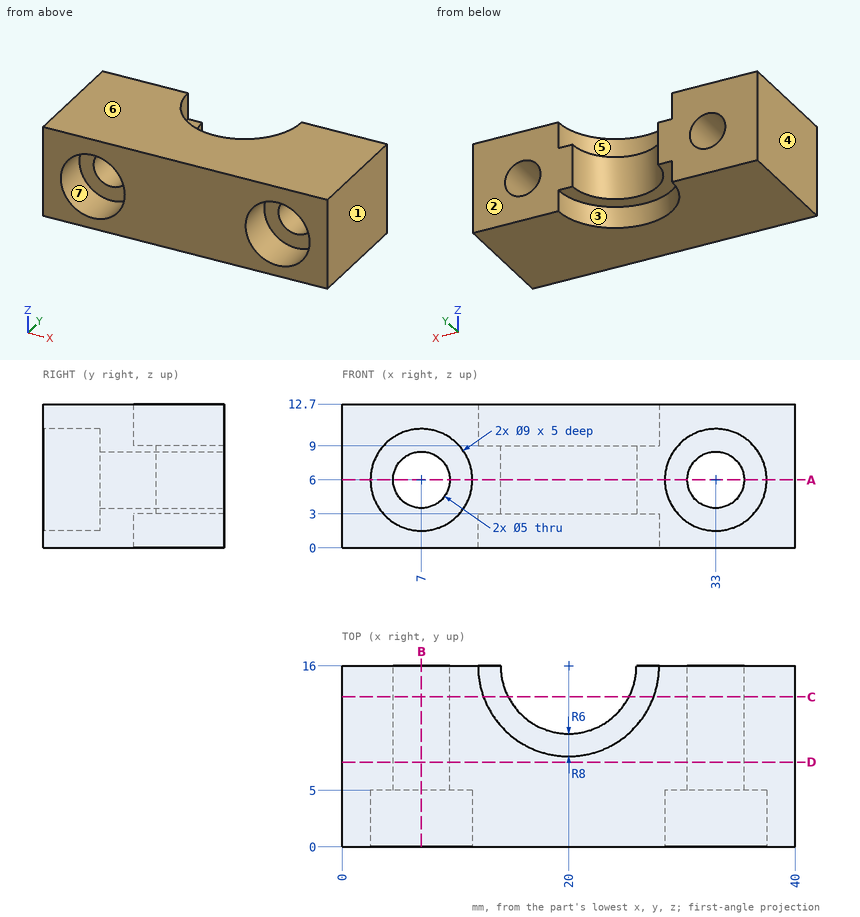
The drawing under review shows one solid part. Ordinate dimensions are in mm from its lowest x, y, z. A direction names the side the tool comes from. Give positions to 0.01 mm unless a question says otherwise; leave off trailing zeros. Order: outer loops, then holes, each group sorted by start corner. A loop starts at its lowest first (then second) coordinate and runs counter-clockwise, first axis right, second up. Notation, with made-up numbers: (60, 36.25) - (81, 36.25) arc R18 cw to (81, 63.25) - close; hole circle Ø3 at (-33.75, 27.25). An arc over 180 degrees is marked (long way). Answer as a JSON object with one key per item and string values. Group by question number.
Item 1: Wall thickness on line 1 along X through (y, z) = (1, 5.75); line 2 along Z through (x, y) = (7, 3.3); line 3 along X through (y, z) = (12.5, 7): over which ranges is each line inside the solid? List them lowest first.
Item 2: Machinability: for the marked faces 5, 6 and 7, which of the approach directions +Z, -Z, +X, -X, +Y, -Y give a long, thin tool a straight path to every point of the face, cutting with its end or side? Answer none if there is none.
Item 3: Clearance check with flat-ended pins moving along their axes: pin 1 Ø2.5 at (x, z) = (6, 7.5) entering from -Y; pin 2 Ø5 at (x, z) = (26, 10.5) entering from -Y; pin 3 Ø2.5 at (x, y) = (19.5, 11) entering from +Z; pin 4 Ø9 at (x, y) = (22, 14) entering from -Z. State where each tip first meets the part, or that it passes through.
Item 4: Take a section at A-A on z = 6. Give the boundary of the cut face in (x, y), and give its area (3 significant figures).
Item 5: Take a section at D-D on y = 7.5. Give the boundary of the cut face in (x, z), and give its area (3 significant figures).
Item 6: Draft analysis for pull direction X (two halves, no side actions). For the marked faces 1, 2, 3 and 4, state which applies: pulls with the +X half, pulls with the -X half, needs draft (parallel to the pull), parting line crosses it, or undercut.
Item 7: Take a section at B-B on x = 7. Give the boundary of the cut face in (y, z).
Item 8: Take a section at C-C on y = 13.25. Give the boundary of the cut face in (x, z), and give its area (3 significant figures).
Reported:
{
 "1": {"line 1": "0 to 2.51, 11.49 to 28.51, 37.49 to 40", "line 2": "0 to 1.5, 10.5 to 12.7", "line 3": "0 to 4.71, 9.29 to 15.13, 24.87 to 30.71, 35.29 to 40"},
 "2": {"face 5": "+Z, +Y", "face 6": "+Z, +X, -X, +Y, -Y", "face 7": "-Y"},
 "3": {"pin 1": "y = 5", "pin 2": "y = 0", "pin 3": "z = 9", "pin 4": "z = 3"},
 "4": {"outline": "(0, 0) - (2.5, 0) - (2.5, 5) - (4.5, 5) - (4.5, 16) - (0, 16) - close; (9.5, 5) - (11.5, 5) - (11.5, 0) - (28.5, 0) - (28.5, 5) - (30.5, 5) - (30.5, 16) - (26, 16) arc R6 cw to (14, 16) - (9.5, 16) - close; (35.5, 5) - (37.5, 5) - (37.5, 0) - (40, 0) - (40, 16) - (35.5, 16) - close", "area": "383 mm^2"},
 "5": {"outline": "(0, 0) - (40, 0) - (40, 12.7) - (0, 12.7) - close; hole circle Ø5 at (7, 6); hole circle Ø5 at (33, 6)", "area": "469 mm^2"},
 "6": {"face 1": "pulls with the +X half", "face 2": "needs draft", "face 3": "undercut", "face 4": "pulls with the -X half"},
 "7": {"outline": "(0, 0) - (16, 0) - (16, 3.5) - (5, 3.5) - (5, 1.5) - (0, 1.5) - close; (0, 10.5) - (5, 10.5) - (5, 8.5) - (16, 8.5) - (16, 12.7) - (0, 12.7) - close"},
 "8": {"outline": "(0, 0) - (12.49, 0) - (12.49, 3) - (14.67, 3) - (14.67, 9) - (12.49, 9) - (12.49, 12.7) - (0, 12.7) - close; (25.33, 3) - (27.51, 3) - (27.51, 0) - (40, 0) - (40, 12.7) - (27.51, 12.7) - (27.51, 9) - (25.33, 9) - close; hole circle Ø5 at (7, 6); hole circle Ø5 at (33, 6)", "area": "304 mm^2"}
}
